The drawing under review shows one solid part. Ordinate dimensions are in mm from its lowest x, y, z. A direction names the side the tool comes from. Give positions to 0.01 mm unless a question says otherwise; leave off trailing zeros. Write each loop counter-clockwise with the first axis right and the second up, starting at its lowest first coordinate (ties: lowest second). Pieces come first, ordered by that corner, then holes.
Q1. Insertion check: P1, Ø2, axis at x = 8.5, z = 2.5, coming from the +Y side; P2, Ø1, axis at y = 3, z = 3.5, coming from the -X side; P3, Ø3, axis at y = 4.5, z = 4, coming from the -X side. Each pin has a flat end and moves straight along its axis. Give the tip position at first contact, or say it passes through.
Q2. We need section D-D (x = 10.5). Write out the cut boundary in (y, z) (3 decimals), then the cut area to 3 significant figures.
Q3. For line 1 (Z direction, x = 0.5, y = 6) (3 decimals); line 2 (Y direction, x = 5.75, z = 1.75); line 3 (X direction, y = 5, z = 1.25), list the stretches that pass through material, from the lowest coordinate up.
Q4. Mouldability with a two-part tool opening along Z and no side actions: class the marked faces 3, 4, 5 and 6 as released by +Z, released by -Z, zero draft, split by the parting line, or undercut.
Q5. We need section A-A (y = 6.35). Write out the cut boundary in (x, z) (3 decimals), then the cut area to 3 significant figures.
Q6. Machinability: for the marked faces 1 and 2, which of the approach directions +Z, -Z, +X, -X, +Y, -Y give a long, thin tool a straight path to every point of the face, cutting with its end or side? Answer none if there is none.
Q7. We need section C-C (z = 3.75). Write out the cut boundary in (x, y).
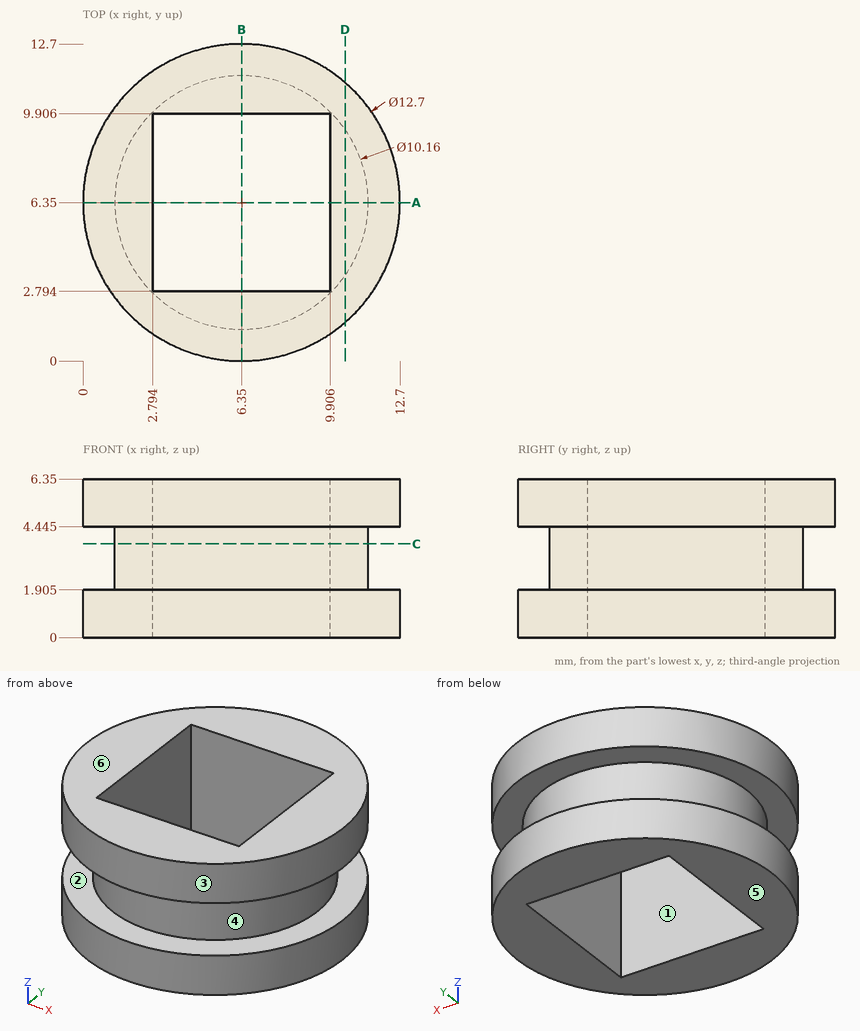
Computed:
1. P1: stops at y = 12.56
1. P2: stops at x = 2.14
1. P3: stops at x = 0.01
2. outline: (1.544, 0) - (11.156, 0) - (11.156, 1.905) - (9.28, 1.905) - (9.28, 4.445) - (11.156, 4.445) - (11.156, 6.35) - (1.544, 6.35) - (1.544, 4.445) - (3.42, 4.445) - (3.42, 1.905) - (1.544, 1.905) - close
2. area: 51.5 mm2
3. line 1: z = 0 to 1.905, 4.445 to 6.35
3. line 2: y = 0.03 to 2.79, 9.91 to 12.67
3. line 3: x = 0.15 to 2.79, 9.91 to 12.55
4. face 3: zero draft
4. face 4: undercut
4. face 5: released by -Z
4. face 6: released by +Z
5. outline: (0, 0) - (2.794, 0) - (2.794, 6.35) - (0, 6.35) - (0, 4.445) - (1.27, 4.445) - (1.27, 1.905) - (0, 1.905) - close; (9.906, 0) - (12.7, 0) - (12.7, 1.905) - (11.43, 1.905) - (11.43, 4.445) - (12.7, 4.445) - (12.7, 6.35) - (9.906, 6.35) - close
5. area: 29.0 mm2
6. face 1: +Z, -Z
6. face 2: none
7. outline: circle Ø10.16 at (6.35, 6.35); hole (2.79, 2.79) - (9.91, 2.79) - (9.91, 9.91) - (2.79, 9.91) - close
